Geometry: see drawing. Coordinates: mm, zero at the bounding-box minimum. A direction names the side the tool comes from. Round coordinates to 2 decimals unless told otherwise and drop trailing zeros. Order: outer loops, then holes, each group sorted by start corner. A loop starts at its lowest first (then second) coordinate and runs counter-clockwise, first axis right, second up. Notation, with made-up numbers: (67, -14.5) -> (113, -14.5) arc R25 cw to (113, 3.5) -> close; hole circle Ø4 at (-28, 33). An arc over 180 degrees is marked (long way). Use a Markdown table: item, result.
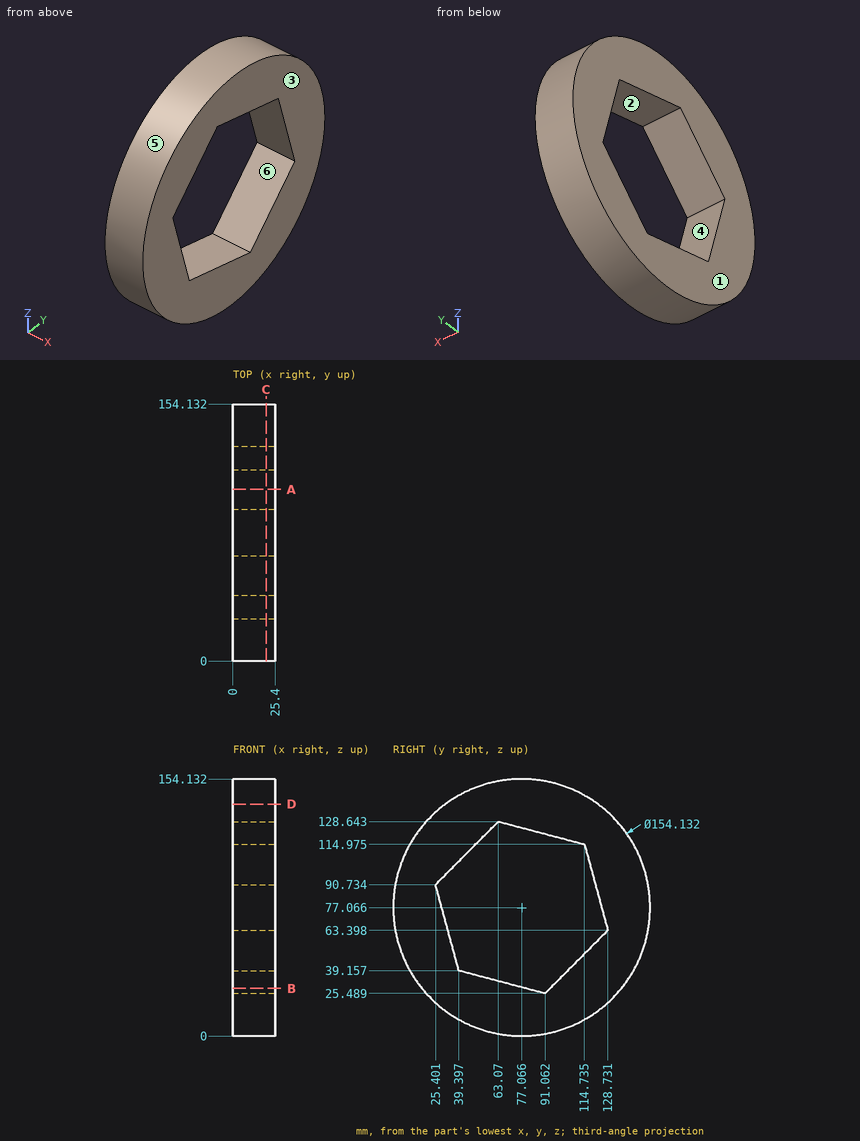
1) Contact query for flat-ended pins moving along their axis: P1, Ø10, axis at x = 15, y = 77.5, coming from the +Z side; P2, Ø8, axis at x = 5.5, y = 23, coming from the -Z side; P3, Ø3, axis at x = 19, y = 84, coming from the -Z side. Output: stop coordinate, or through.
Answer key:
| item | result |
|---|---|
| P1 | stops at z = 154.13 |
| P2 | stops at z = 18.48 |
| P3 | stops at z = 0.19 |
2) Cut plane A-A on y = 103. Return loops of the section in (x, z) (1 decimal), and give its area (3 significant figures).
Answer key:
| item | result |
|---|---|
| outline | (0, 4.5) -> (25.4, 4.5) -> (25.4, 37.5) -> (0, 37.5) -> close; (0, 118.1) -> (25.4, 118.1) -> (25.4, 149.6) -> (0, 149.6) -> close |
| area | 1,640 mm^2 |
3) Set-up query: the marked faces 1 and 2. Return all of +Z, -Z, +X, -X, +Y, -Y with unobstructed straight access to the full face (end or side cutting, diameter ignored); none if empty.
Answer key:
| item | result |
|---|---|
| face 1 | +Z, -Z, -X, +Y, -Y |
| face 2 | +X, -X |
4) Draft query along Z for the marked faces 3, 4, 5 and 6. Return one class per face: released by +Z, released by -Z, zero draft, split by the parting line, or undercut.
Answer key:
| item | result |
|---|---|
| face 3 | zero draft |
| face 4 | undercut |
| face 5 | split by the parting line |
| face 6 | undercut |
5) Cut plane D-D on z = 139. Return loops of the section in (x, y), and give its area (3 significant figures).
Answer key:
| item | result |
|---|---|
| outline | (0, 31.2) -> (25.4, 31.2) -> (25.4, 122.93) -> (0, 122.93) -> close |
| area | 2,330 mm^2 |
6) Cut plane B-B on z = 28.5. Return loops of the section in (x, y), and give its area (3 significant figures).
Answer key:
| item | result |
|---|---|
| outline | (0, 17.23) -> (25.4, 17.23) -> (25.4, 79.68) -> (0, 79.68) -> close; (0, 94.05) -> (25.4, 94.05) -> (25.4, 136.9) -> (0, 136.9) -> close |
| area | 2,670 mm^2 |
7) Ray query, probe 1 along Y at (x, z) = (3.25, 75) (1 decimal); probe 2 along Y at (x, z) = (11, 106) (1 decimal); probe 3 along Z at (x, y) = (8.5, 50.5) (1 decimal). Return the intervals inside material, ascending.
Answer key:
| item | result |
|---|---|
| probe 1 | y = 0 to 29.7, 125.6 to 154.1 |
| probe 2 | y = 5.6 to 40.6, 117.2 to 148.5 |
| probe 3 | z = 4.7 to 36.2, 116 to 149.4 |
8) Cut plane C-C on x = 20. Return loops of the section in (y, z) (1 decimal), and give its area (3 significant figures).
Answer key:
| item | result |
|---|---|
| outline | circle Ø154.1 at (77.1, 77.1); hole (25.4, 90.7) -> (39.4, 39.2) -> (91.1, 25.5) -> (128.7, 63.4) -> (114.7, 115) -> (63.1, 128.6) -> close |
| area | 11,200 mm^2 |
